Geometry: see drawing. Coordinates: mm, zero at the bounding-box minimum. Coordinates: 2 decimals unless noted, no trailing zeros. Write each loop counter-clockwise with the first axis right and the second up, starting at its lowest first coordinate (ties: lowest second). Pieces come first, ordered by that corner, then holes. Notation, with made-up numbers: M 71,28 L 75,28 A24 cw 75,57 Z; hole C 69.5,69 d3. An arc over 180 degrees is marked long. One line per item, written item: value. Start each with the question number.
Item 1: Cut plane C-C, the plane x = 79. Output: boundary loops of the cut face in (y, z).
Item 2: Cut plane A-A, the plane z = 6.25. Output: boundary loops of the cut face in (x, y), then the cut area to 3 significant figures.
Item 3: Cut plane B-B, the plane y = 512.1. Output: boundary loops of the cut face in (x, z), then the cut area to 3 significant figures.
Item 4: Pin query (flat end, axial travel): P1, Ø1.5, axis at x = 72, z = 7, coming from the -Y side. Return the tip coordinate at first contact, or that it passes through.
Item 5: Ray query, L1, parallel to Y at x = 50, z = 5.75; L2, parallel to Y at x = 15, z = 6.5; L3, parallel to Y at x = 47, z = 2.25. Return the intervals inside material, ascending. Write a range as from..to.
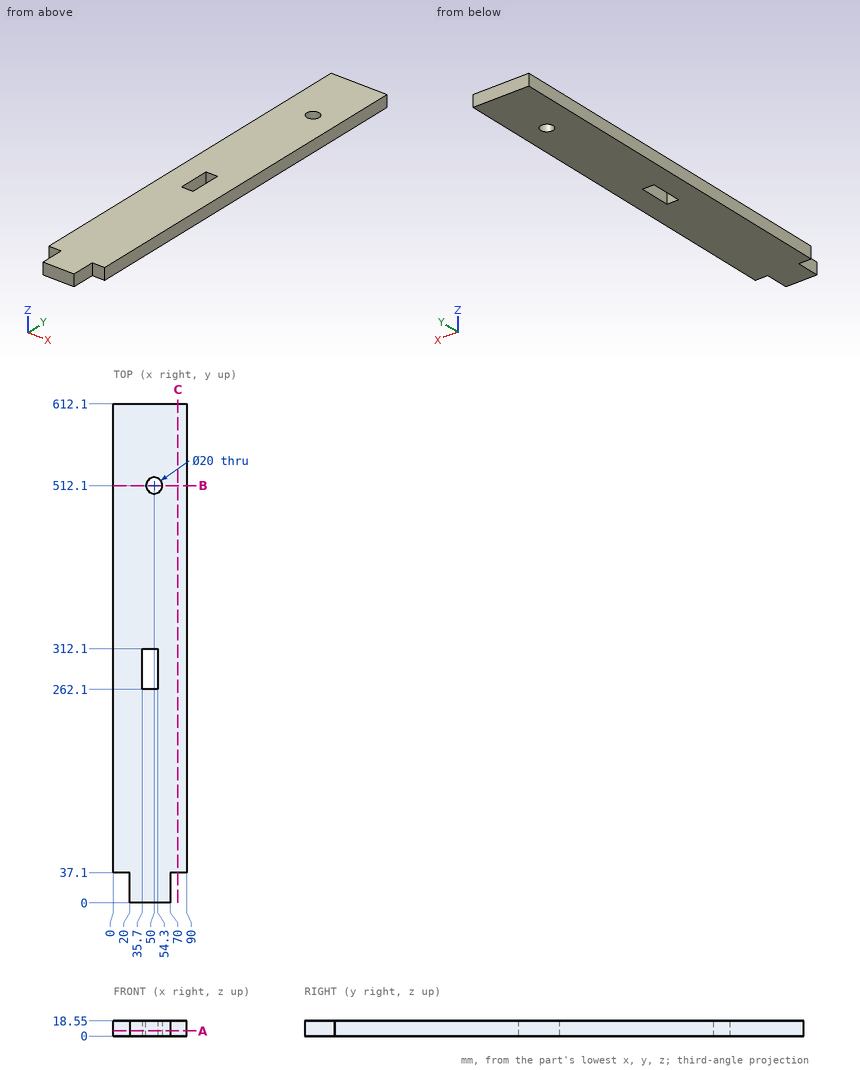
From the geometry:
1. outline: M 37.1,0 L 612.1,0 L 612.1,18.55 L 37.1,18.55 Z
2. outline: M 0,37.1 L 20,37.1 L 20,0 L 70,0 L 70,37.1 L 90,37.1 L 90,612.1 L 0,612.1 Z; hole M 35.7,262.1 L 54.3,262.1 L 54.3,312.1 L 35.7,312.1 Z; hole C 50,512.1 d20
2. area: 52,400 mm²
3. outline: M 0,0 L 40,0 L 40,18.55 L 0,18.55 Z; M 60,0 L 90,0 L 90,18.55 L 60,18.55 Z
3. area: 1,300 mm²
4. P1: stops at y = 37.1
5. L1: y = 0..262.1, 312.1..502.1, 522.1..612.1
5. L2: y = 37.1..612.1
5. L3: y = 0..262.1, 312.1..502.56, 521.64..612.1
